Build history of the part. All positions in model axes, mm. Face numbers are marked on the shaded views. A direction names the side the tool comes from. Coordinates: 2 decimals unless noted, no trailing zeros. Order: outer loops, then holes, each group sorted by start corner. A loop starts at its lowest first (then second) coordinate and runs counter-clockwise, first axis right, second up. Notation, with made-up numbers: (-36, 9) - (-29, 9) arc R33 cw to (-29, 40) - close; hole circle Ø1 at (25.25, 43.25). An arc over 180 degrees is marked (long way). Return JSON: item names as keys, results as strings.
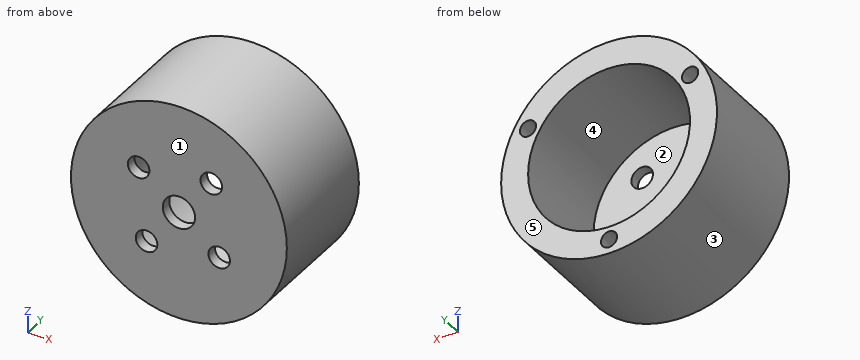
from build123d import *

# Parameters (mm, degrees)
SKETCH1_R           = 20
SKETCH1_R_2         = 15
BOSS_EXTRUDE1_DEPTH = 20
SKETCH2_R           = 20
SKETCH2_R_2         = 3
SKETCH2_R_3         = 2
BOSS_EXTRUDE2_DEPTH = 2
SKETCH3_R           = 1.5
CUT_EXTRUDE1_DEPTH  = 4


with BuildPart() as part:
    # Sketch1 → Boss-Extrude1 (new body)
    with BuildSketch(Plane(origin=(0, 0, 0), x_dir=(1, 0, 0), z_dir=(0, 1, 0))):
        Circle(SKETCH1_R)
        Circle(SKETCH1_R_2, mode=Mode.SUBTRACT)
    extrude(amount=BOSS_EXTRUDE1_DEPTH)

    # Sketch2 → Boss-Extrude2 (add)
    with BuildSketch(Plane.XZ):
        Circle(SKETCH2_R)
        Circle(SKETCH2_R_2, mode=Mode.SUBTRACT)
        with Locations((6, 7.463372557)):
            Circle(SKETCH2_R_3, mode=Mode.SUBTRACT)
        with Locations((7.463372557, -6)):
            Circle(SKETCH2_R_3, mode=Mode.SUBTRACT)
        with Locations((-6, -7.463372557)):
            Circle(SKETCH2_R_3, mode=Mode.SUBTRACT)
        with Locations((-7.463372557, 6)):
            Circle(SKETCH2_R_3, mode=Mode.SUBTRACT)
    extrude(amount=BOSS_EXTRUDE2_DEPTH)

    # Sketch3 → Cut-Extrude1 (cut)
    with BuildSketch(Plane(origin=(0, 20, 0), x_dir=(1, 0, 0), z_dir=(0, 1, 0))):
        with Locations((0, 17.343709181)):
            Circle(SKETCH3_R)
        with Locations((15.020092746, -8.67185459)):
            Circle(SKETCH3_R)
        with Locations((-15.020092746, -8.67185459)):
            Circle(SKETCH3_R)
    extrude(amount=-CUT_EXTRUDE1_DEPTH, mode=Mode.SUBTRACT)


solid = part.part
1. Probe L1, parallel to Z at x = 0, y = 17; L2, parallel to Z at x = -6, y = -0.9; L3, parallel to Y at x = 1.5, z = 4. List the from-to ranges inside material, lowest first.
Check values:
{"L1": "-20 to -18.84, -15.84 to -15, 15 to 20", "L2": "-19.08 to -9.46, -5.46 to 4.64, 7.36 to 19.08", "L3": "-2 to 0"}
2. Cut at C-C on y = 11. Give the cut face in (x, z), plus the area to 3 significant figures.
Check values:
{"outline": "circle Ø40 at (0, 0); hole circle Ø30 at (0, 0)", "area": "550 mm²"}
3. Drop flat-ended pins along their axis: pin 1 (3.5 mm diameter, centred on x = 6, z = 7.46, fed in from +Y); pin 2 (5 mm diameter, centred on x = 6, y = 5, fed in from -Z); pin 3 (2 mm diameter, centred on x = -5.5, y = 9, fed in from +Z); pin 4 (1.5 mm diameter, centred on y = 16.5, z = 14, fed in from +X). Give the stop position or say it passes through.
Check values:
{"pin 1": "through", "pin 2": "z = -19.69", "pin 3": "z = 19.49", "pin 4": "x = 14.98"}
4. Mould opens along Z. For the marked faces 3, 4 and 5 say: pulls with the +Z half, pulls with the -Z half, needs draft (parallel to the pull), parting line crosses it, or undercut.
Check values:
{"face 3": "parting line crosses it", "face 4": "undercut", "face 5": "needs draft"}
5. Cut at B-B on x = 0. Give the cut face in (y, z), plus the area to 3 significant figures.
Check values:
{"outline": "(-2, -20) - (20, -20) - (20, -18.84) - (16, -18.84) - (16, -15.84) - (20, -15.84) - (20, -15) - (0, -15) - (0, -3) - (-2, -3) - close; (-2, 3) - (0, 3) - (0, 15) - (20, 15) - (20, 20) - (-2, 20) - close", "area": "256 mm²"}
6. Cut at D-D on x = -12. Give the cut face in (y, z).
Check values:
{"outline": "(-2, -16) - (20, -16) - (20, -9) - (0, -9) - (0, 9) - (20, 9) - (20, 16) - (-2, 16) - close"}
7. Cut at A-A on z = 0. Give the cut face in (x, y).
Check values:
{"outline": "(-20, -2) - (-3, -2) - (-3, 0) - (-15, 0) - (-15, 20) - (-20, 20) - close; (3, -2) - (20, -2) - (20, 20) - (15, 20) - (15, 0) - (3, 0) - close"}
8. Tool access for the marked faces 1 and 2: list every direction of +Z, -Z, +X, -X, +Y, -Y with a clear straight run to the whole face (end or side of a thin tool).
Check values:
{"face 1": "+Z, -Z, +X, -X, -Y", "face 2": "+Y"}
